Geometry check sheet. Reference: the model listing, model coordinates, mm. Face numbers are marked on the shaded views. A direction names the side the tool comes from. Give positions to 0.01 mm unless a question says otherwise; leave off trailing zeros. Loops run counter-clockwise (first coordinate to the right, second up) from the corner with the lowest first, then second, coordinate; pieces in that order, holes last.
```python
from build123d import *

# Parameters (mm, degrees)
SKETCH1_R           = 35
BOSS_EXTRUDE1_DEPTH = 6
SKETCH2_R           = 3.75
CUT_EXTRUDE1_DEPTH  = 4
SKETCH3_R           = 6
SKETCH3_R_2         = 2.5
CUT_EXTRUDE2_DEPTH  = 50.859803449
SKETCH4_R           = 35
SKETCH4_R_2         = 30
BOSS_EXTRUDE2_DEPTH = 7
SKETCH5_R           = 30
SKETCH5_R_2         = 26
BOSS_EXTRUDE3_DEPTH = 7
SKETCH6_R           = 1.75
CUT_EXTRUDE3_DEPTH  = 52.176166328
SKETCH7_R           = 2
CUT_EXTRUDE4_DEPTH  = 3


with BuildPart() as part:
    # Sketch1 → Boss-Extrude1 (new body)
    with BuildSketch(Plane(origin=(0, 0, 0), x_dir=(1, 0, 0), z_dir=(0, 1, 0))):
        with Locations(Location((0, 0, 0), (0, 0, 270))):
            Circle(SKETCH1_R)
    extrude(amount=BOSS_EXTRUDE1_DEPTH)

    # Sketch2 → Cut-Extrude1 (cut)
    with BuildSketch(Plane(origin=(0, 6, 0), x_dir=(1, 0, 0), z_dir=(0, 1, 0))):
        with Locations(Location((0, 21, 0), (0, 0, 270))):
            Circle(SKETCH2_R)
        with Locations(Location((21, 0, 0), (0, 0, 270))):
            Circle(SKETCH2_R)
        with Locations(Location((0, -21, 0), (0, 0, 270))):
            Circle(SKETCH2_R)
        with Locations(Location((-21, 0, 0), (0, 0, 270))):
            Circle(SKETCH2_R)
    extrude(amount=-CUT_EXTRUDE1_DEPTH, mode=Mode.SUBTRACT)

    # Sketch3 → Cut-Extrude2 (cut, through all)
    with BuildSketch(Plane(origin=(0, 6, 0), x_dir=(1, 0, 0), z_dir=(0, 1, 0))):
        with Locations(Location((0, 0, 0), (0, 0, 270))):
            Circle(SKETCH3_R)
        with Locations(Location((0, 21, 0), (0, 0, 270))):
            Circle(SKETCH3_R_2)
        with Locations(Location((21, 0, 0), (0, 0, 270))):
            Circle(SKETCH3_R_2)
        with Locations(Location((0, -21, 0), (0, 0, 270))):
            Circle(SKETCH3_R_2)
        with Locations(Location((-21, 0, 0), (0, 0, 270))):
            Circle(SKETCH3_R_2)
    extrude(amount=-CUT_EXTRUDE2_DEPTH, mode=Mode.SUBTRACT)

    # Sketch4 → Boss-Extrude2 (add)
    with BuildSketch(Plane(origin=(0, 6, 0), x_dir=(1, 0, 0), z_dir=(0, 1, 0))):
        with Locations(Location((0, 0, 0), (0, 0, 270))):
            Circle(SKETCH4_R)
        with Locations(Location((0, 0, 0), (0, 0, 270))):
            Circle(SKETCH4_R_2, mode=Mode.SUBTRACT)
    extrude(amount=BOSS_EXTRUDE2_DEPTH)

    # Sketch5 → Boss-Extrude3 (add)
    with BuildSketch(Plane(origin=(0, 6, 0), x_dir=(1, 0, 0), z_dir=(0, 1, 0))):
        Circle(SKETCH5_R)
        with Locations(Location((0, 0, 0), (0, 0, 270))):
            Circle(SKETCH5_R_2, mode=Mode.SUBTRACT)
    extrude(amount=BOSS_EXTRUDE3_DEPTH)

    # Sketch6 → Cut-Extrude3 (cut, through all)
    with BuildSketch(Plane(origin=(0, 13, 0), x_dir=(1, 0, 0), z_dir=(0, 1, 0))):
        with Locations(Location((0, 32.5, 0), (0, 0, 270))):
            Circle(SKETCH6_R)
        with Locations(Location((32.5, 0, 0), (0, 0, 270))):
            Circle(SKETCH6_R)
        with Locations(Location((0, -32.5, 0), (0, 0, 270))):
            Circle(SKETCH6_R)
        with Locations(Location((-32.5, 0, 0), (0, 0, 270))):
            Circle(SKETCH6_R)
    extrude(amount=-CUT_EXTRUDE3_DEPTH, mode=Mode.SUBTRACT)

    # Sketch7 → Cut-Extrude4 (cut)
    with BuildSketch(Plane.XZ):
        with Locations(Location((0, 32.5, 0), (0, 0, 270))):
            Circle(SKETCH7_R)
        with Locations(Location((32.5, 0, 0), (0, 0, 270))):
            Circle(SKETCH7_R)
        with Locations(Location((0, -32.5, 0), (0, 0, 270))):
            Circle(SKETCH7_R)
        with Locations(Location((-32.5, 0, 0), (0, 0, 270))):
            Circle(SKETCH7_R)
    extrude(amount=-CUT_EXTRUDE4_DEPTH, mode=Mode.SUBTRACT)


solid = part.part
```
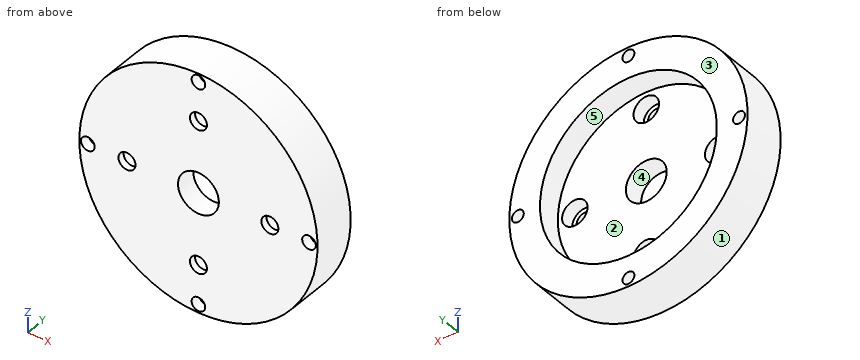
1) Sectioned sample at A-A on x = -32.5. Enter the section's corners in (y, z), plus the area to 3 significant figures.
2) Sectioned sample at B-B on z = 21. Enter the section's corners in (x, y).
3) Depth check by flat-ended pin: P1, Ø5, axis at x = -25.5, y = 2.5, coming from the +Z side; P2, Ø3, axis at x = -32.5, z = 0, coming from the -Y side; P3, Ø4, axis at y = 8.5, z = -19, coming from the +X side; P4, Ø6, axis at x = -22, z = 2, coming from the +Y side. Enter the tip coordinate at first touch or a pass-through.
4) Tool access check on the marked faces 4 and 5. Record the directions out of +Z, -Z, +X, -X, +Y, -Y that give a thin tool (end or side, any length) a straight path to the whole face; none if there is none.
5) Sectioned sample at D-D on z = 0. Count the separate pieces of the cut face and the enclosed holes in it, plus the area to 3 significant figures.
6) Mould release check, pull along X, two halves, no side actions. Record for the marked faces 1, 2 and 3: +X half, -X half, draft (parallel to the pull), parting line (faces both ways), or undercut.
7) Sectioned sample at C-C on y = 7.25. Enter the section's corners in (x, z).
8) Scan lines: line 1 along X through (y, z) = (1.15, 0); line 2 along X through (y, z) = (2.4, 0); line 3 along Y through (x, z) = (-6.5, 19). Record each from-to range of solid material in increasing order.
Determined:
1. outline: (0, -12.99) - (13, -12.99) - (13, -1.75) - (3, -1.75) - (3, -2) - (0, -2) - close; (0, 2) - (3, 2) - (3, 1.75) - (13, 1.75) - (13, 12.99) - (0, 12.99) - close
1. area: 291 mm2
2. outline: (-28, 0) - (-2.5, 0) - (-2.5, 2) - (-3.75, 2) - (-3.75, 6) - (-15.33, 6) - (-15.33, 13) - (-28, 13) - close; (2.5, 0) - (28, 0) - (28, 13) - (15.33, 13) - (15.33, 6) - (3.75, 6) - (3.75, 2) - (2.5, 2) - close
3. P1: stops at z = 26.38
3. P2: passes through
3. P3: stops at x = 30.59
3. P4: stops at y = 6
4. face 4: +Y, -Y
4. face 5: +Y
5. separate pieces: 6
5. enclosed holes: 0
5. area: 300 mm2
6. face 1: parting line
6. face 2: undercut
6. face 3: draft
7. outline: circle Ø70 at (0, 0); hole circle Ø3.5 at (-32.5, 0); hole circle Ø52 at (0, 0); hole circle Ø3.5 at (0, -32.5); hole circle Ø3.5 at (0, 32.5); hole circle Ø3.5 at (32.5, 0)
8. line 1: x = -35 to -34.5, -30.5 to -23.5, -18.5 to -6, 6 to 18.5, 23.5 to 30.5, 34.5 to 35
8. line 2: x = -35 to -34.5, -30.5 to -24.75, -17.25 to -6, 6 to 17.25, 24.75 to 30.5, 34.5 to 35
8. line 3: y = 0 to 6
